Part model, mm, in its own coordinate system. Round coordinates to 2 decimals unless told otherwise and drop trailing zeros. Return JSON: item names as keys, results as strings. Group by question number.
Item 1: Saw through at A-A on x = -152.5. State how many separate pieces and enclosed holes the cut face has, and give its area (3 significant figures).
Item 2: Drop flat-ended pins along their axis: pin 1 (2 mm diameter, centred on x = -127.5, z = -2.5, fed in from -Y); pin 2 (1.9 mm diameter, centred on x = 27.5, z = -12, fed in from -Y); pin 3 (1.7 mm diameter, centred on x = -66.5, z = 5.5, fed in from -Y). Give the stop position or say it passes through.
Item 3: Probe probe 1 along Z at (x, y) = (202.5, 11.25); probe 2 along Z at (x, y) = (100, 2.25); probe 3 along Y at (x, z) = (-108, 0). List the from-to ranges inside material, lowest first.
Item 4: Two-plate mould, pull along Z, no slides. Class faces 1 (the face through (3.47, -5.11, 4.82)), 2 (the face through (247.65, 3, 0)), 3 (the face through (3.47, -7.27, 6.97)): released by +Z, released by -Z, zero draft, split by the parting line, or undercut.
```python
from build123d import *

# Parameters (mm, degrees)
SKETCH3_R                = 2.5527
BOSS_EXTRUDE1_DEPTH      = 247.65
BOSS_EXTRUDE1_DEPTH_BACK = 247.65


with BuildPart() as part:
    # Sketch3 → Boss-Extrude1 (new body, two sides)
    with BuildSketch(Plane(origin=(0, 0, 0), x_dir=(0, 0, -1), z_dir=(1, 0, 0))) as boss_extrude1_sk:
        with BuildLine():
            Line((-10.668, 12.7), (-3.2385, 12.7))
            Line((-3.2385, 12.7), (-3.2385, 10.3632))
            Line((-3.2385, 10.3632), (-8.800635435, 10.3632))
            Line((-8.800635435, 10.3632), (-3.187235669, 4.749800235))
            Line((-3.187235669, 4.749800235), (3.187235669, 4.749800235))
            Line((3.187235669, 4.749800235), (8.800635435, 10.3632))
            Line((8.800635435, 10.3632), (3.2385, 10.3632))
            Line((3.2385, 10.3632), (3.2385, 12.7))
            Line((3.2385, 12.7), (10.668, 12.7))
            ThreePointArc((10.668, 12.7), (12.104840979, 12.104840979), (12.7, 10.668))
            Line((12.7, 10.668), (12.7, 3.2385))
            Line((12.7, 3.2385), (10.3632, 3.2385))
            Line((10.3632, 3.2385), (10.3632, 8.800635435))
            Line((10.3632, 8.800635435), (4.749800235, 3.187235669))
            Line((4.749800235, 3.187235669), (4.749800235, -3.187235669))
            Line((4.749800235, -3.187235669), (10.3632, -8.800635435))
            Line((10.3632, -8.800635435), (10.3632, -3.2385))
            Line((10.3632, -3.2385), (12.7, -3.2385))
            Line((12.7, -3.2385), (12.7, -10.668))
            ThreePointArc((12.7, -10.668), (12.104840979, -12.104840979), (10.668, -12.7))
            Line((10.668, -12.7), (6.35, -12.7))
            ThreePointArc((6.35, -12.7), (-7.120384182, -7.120384182), (-12.7, 6.35))
            Line((-12.7, 6.35), (-12.7, 10.668))
            ThreePointArc((-12.7, 10.668), (-12.104840979, 12.104840979), (-10.668, 12.7))
        make_face()
        Circle(SKETCH3_R, mode=Mode.SUBTRACT)
        with BuildLine():
            Line((2.485198871, -4.047763436), (8.003751298, -9.566315863))
            ThreePointArc((8.003751298, -9.566315863), (-4.965122713, -4.965122713), (-9.566315863, 8.003751298))
            Line((-9.566315863, 8.003751298), (-4.047763436, 2.485198871))
            ThreePointArc((-4.047763436, 2.485198871), (-3.358615955, -3.358615955), (2.485198871, -4.047763436))
        make_face(mode=Mode.SUBTRACT)
    extrude(amount=BOSS_EXTRUDE1_DEPTH)
    extrude(boss_extrude1_sk.sketch, amount=-BOSS_EXTRUDE1_DEPTH_BACK)


solid = part.part
```
Filled in:
{
 "1": {"separate pieces": "1", "enclosed holes": "2", "area": "302 mm^2"},
 "2": {"pin 1": "stops at y = -12.49", "pin 2": "stops at y = -12.66", "pin 3": "stops at y = -9.2"},
 "3": {"probe 1": "z = -12.61 to -3.24, 3.24 to 12.61", "probe 2": "z = -4.75 to -1.21, 1.21 to 4.18, 9.12 to 12.25", "probe 3": "y = -11.61 to -8.34, -4.75 to -2.55, 2.55 to 4.75"},
 "4": {"face 1": "undercut", "face 2": "zero draft", "face 3": "released by +Z"}
}
